from build123d import *

# Parameters (mm, degrees)
F1_DEPTH = 22.5
F3_START = 12
F2_R     = 2.5
F3_DEPTH = 13


with BuildPart() as f1:
    # F0 (on Front) → F1 (new body, symmetric)
    with BuildSketch(Plane.XZ):
        with BuildLine():
            Line((22.5, 6.23), (22.5, 16.5))
            Line((22.5, 16.5), (-22.5, 16.5))
            Line((-22.5, 16.5), (-22.5, 6.23))
            Line((-22.5, 6.23), (-21.23, 6.23))
            Line((-21.23, 6.23), (-21.23, -16.5))
            Line((-21.23, -16.5), (-10.53, -16.5))
            Line((-10.53, -16.5), (-5.0353739326, -9.7165110278))
            ThreePointArc((-5.0353739326, -9.7165110278), (0, 4.5), (5.0353739326, -9.7165110278))
            Line((5.0353739326, -9.7165110278), (10.53, -16.5))
            Line((10.53, -16.5), (21.23, -16.5))
            Line((21.23, -16.5), (21.23, 6.23))
            Line((21.23, 6.23), (22.5, 6.23))
        make_face()
    extrude(amount=F1_DEPTH, both=True)

    # F2 (on Top) → F3 (cut)
    with BuildSketch(Plane.XY.offset(F3_START)):
        with Locations((-16, 15)):
            Circle(F2_R)
        with Locations((-16, -15)):
            Circle(F2_R)
        with Locations((16, 15)):
            Circle(F2_R)
        with Locations((16, -15)):
            Circle(F2_R)
    extrude(amount=F3_DEPTH, mode=Mode.SUBTRACT)


solid = f1.part
Could you check a few things on this model? Use its own coordinates, in mm. A direction names the side the tool comes from. Give positions to 0.01 mm unless a question says otherwise; leave off trailing zeros. Loops run counter-clockwise (first coordinate to the right, second up) from the corner with the lowest first, then second, coordinate; pieces in that order, holes last. Notation, with made-up numbers: (37, -25.75) -> (43, -25.75) arc R22 ccw to (43, -5.75) -> close; hole circle Ø5 at (20, -14). An arc over 180 degrees is marked (long way). Return JSON: item names as keys, results as strings.
Item 1: I'm going to push flat-ended pins straight in: pin 1 (1 mm diameter, centred on x = -22, y = 4.5, fed in from -Z); pin 2 (1.5 mm diameter, centred on x = 15, y = -15.5, fed in from +Z); pin 3 (14.5 mm diameter, centred on x = 0, z = -3.5, fed in from +Y); pin 4 (4 mm diameter, centred on y = 3, z = -8, fed in from -X). Where does each tip first touch, or does it pass through?
Geometry results:
{"pin 1": "stops at z = 6.23", "pin 2": "stops at z = 12", "pin 3": "passes through", "pin 4": "stops at x = -21.23"}
Item 2: If we section it at B-B on x = 16: List the corners of the cut face in (y, z) for me, plus the area to 3 significant figures.
Geometry results:
{"outline": "(-22.5, -16.5) -> (22.5, -16.5) -> (22.5, 16.5) -> (17.5, 16.5) -> (17.5, 12) -> (12.5, 12) -> (12.5, 16.5) -> (-12.5, 16.5) -> (-12.5, 12) -> (-17.5, 12) -> (-17.5, 16.5) -> (-22.5, 16.5) -> close", "area": "1,440 mm²"}
Item 3: If we section it at A-A on z = -3.5: List the corners of the cut face in (x, y) for me.
Geometry results:
{"outline": "(-21.23, -22.5) -> (-8, -22.5) -> (-8, 22.5) -> (-21.23, 22.5) -> close; (8, -22.5) -> (21.23, -22.5) -> (21.23, 22.5) -> (8, 22.5) -> close"}
Item 4: If we section it at D-D on y = 20.5: List the corners of the cut face in (x, z) for me.
Geometry results:
{"outline": "(-22.5, 6.23) -> (-21.23, 6.23) -> (-21.23, -16.5) -> (-10.53, -16.5) -> (-5.04, -9.72) arc R8 cw (long way) to (5.04, -9.72) -> (10.53, -16.5) -> (21.23, -16.5) -> (21.23, 6.23) -> (22.5, 6.23) -> (22.5, 16.5) -> (-22.5, 16.5) -> close"}
Item 5: I need wall thicknesses on L1, parallel to Y at x = 16, z = 13.4; L2, parallel to X at y = 15, z = 14; L3, parallel to Z at x = 16.5, y = -15. Which ranges of each line are inside material? Lowest first, please. Write a range as from..to.
Geometry results:
{"L1": "y = -22.5..-17.5, -12.5..12.5, 17.5..22.5", "L2": "x = -22.5..-18.5, -13.5..13.5, 18.5..22.5", "L3": "z = -16.5..12"}
Item 6: Which directions (+Z, -Z, +X, -X, +Y, -Y) give clear straight access to the entire face, cutting with the end or side of a thin tool? Please do faces 4 (the flat face through (7.744, -0.315, -13.061)), 5 (the flat face through (-21.23, 0, -5)), 6 (the cylindrical face through (-18, 13.5, 14.2)).
Geometry results:
{"face 4": "-Z, +Y, -Y", "face 5": "-Z, -X, +Y, -Y", "face 6": "+Z"}
Item 7: If we section it at C-C on y = -15: List the corners of the cut face in (x, z) for me.
Geometry results:
{"outline": "(-22.5, 6.23) -> (-21.23, 6.23) -> (-21.23, -16.5) -> (-10.53, -16.5) -> (-5.04, -9.72) arc R8 cw (long way) to (5.04, -9.72) -> (10.53, -16.5) -> (21.23, -16.5) -> (21.23, 6.23) -> (22.5, 6.23) -> (22.5, 16.5) -> (18.5, 16.5) -> (18.5, 12) -> (13.5, 12) -> (13.5, 16.5) -> (-13.5, 16.5) -> (-13.5, 12) -> (-18.5, 12) -> (-18.5, 16.5) -> (-22.5, 16.5) -> close"}
Item 8: We'd pull the mould along Y, two halves only. Please class faces 1 (the flat face through (16, -15, 12)), 2 (the flat face through (-22, 0, 6.23)), 3 (the flat face through (-5, -22.5, 4)): +Y half, -Y half, draft (parallel to the pull), parting line (faces both ways), or undercut.
Geometry results:
{"face 1": "undercut", "face 2": "draft", "face 3": "-Y half"}
